Source: CAD feature listing. Evaluate the final solid. Frame: model axes, mm. Face numbers are marked on the shaded views. Coordinates: 2 decimals unless noted, no trailing zeros. Loops run counter-clockwise (first coordinate to the right, second up) from the corner with the lowest first, then second, coordinate; pieces in that order, holes last.
Item 1: Line query: probe 1 along Z at (x, y) = (0, -0.45); probe 2 along Z at (x, y) = (0, 78); probe 3 along Y at (x, z) = (20, 30.5). Output: solid intervals per line, ascending.
Item 2: Pull-direction query (Y, two-part tool) for the marked faces 1, 2 and 3; classes: +Y half, -Y half, draft (parallel to the pull), parting line (faces both ways), or undercut.
Item 3: Pin query (flat end, axial travel): pin 1 Ø12 at (x, z) = (-7, -14.5) entering from +Y; pin 2 Ø5 at (x, y) = (17, 91) entering from +Z; pin 3 Ø3 at (x, y) = (-14, 119) entering from +Z; pin 4 Ø1.5 at (y, z) = (69, -17) entering from +X. Return the tip coordinate at first contact, or that it passes through.
Item 4: Section query A-A, the plane z = 0. Return the cut outline in (x, y).
Item 5: Section query B-B, the plane x = 0. Return the cut outline in (y, z).
Item 6: Section query D-D, the plane x = 33. Return the cut outline in (y, z), then the cut area to 3 significant figures.
Item 7: Section query C-C, the plane y = 74. Return the cut outline in (x, z), then the cut area to 3 significant figures.
```python
from build123d import *

# Parameters (mm, degrees)
F0_R     = 40
F0_R_2   = 28
F0_R_3   = 25.5
F1_DEPTH = 2.5
F2_DEPTH = 160


with BuildPart() as f1:
    # F0 (on Front) → F1 (new body)
    with BuildSketch(Plane.XZ):
        Circle(F0_R)
        with BuildLine():
            ThreePointArc((24.4501319139, 21.4112365218), (30.4210394892, 11.4372355226), (32.5, 0))
            ThreePointArc((32.5, 0), (30.4210394892, -11.4372355226), (24.4501319139, -21.4112365218))
            ThreePointArc((24.4501319139, -21.4112365218), (24.9534304363, -22.1254580507), (25.1309703886, -22.9809703886))
            ThreePointArc((25.1309703886, -22.9809703886), (23.7707716884, -24.9806488394), (21.4112365218, -24.4501319139))
            ThreePointArc((21.4112365218, -24.4501319139), (0, -32.5), (-21.4112365218, -24.4501319139))
            ThreePointArc((-21.4112365218, -24.4501319139), (-24.5012499681, -24.5012499681), (-24.4501319139, -21.4112365218))
            ThreePointArc((-24.4501319139, -21.4112365218), (-32.5, 0), (-24.4501319139, 21.4112365218))
            ThreePointArc((-24.4501319139, 21.4112365218), (-24.5012499681, 24.5012499681), (-21.4112365218, 24.4501319139))
            ThreePointArc((-21.4112365218, 24.4501319139), (0, 32.5), (21.4112365218, 24.4501319139))
            ThreePointArc((21.4112365218, 24.4501319139), (23.7707716884, 24.9806488394), (25.1309703886, 22.9809703886))
            ThreePointArc((25.1309703886, 22.9809703886), (24.9534304363, 22.1254580507), (24.4501319139, 21.4112365218))
        make_face(mode=Mode.SUBTRACT)
        with BuildLine():
            ThreePointArc((24.4501319139, -21.4112365218), (30.4210394892, -11.4372355226), (32.5, 0))
            ThreePointArc((32.5, 0), (30.4210394892, 11.4372355226), (24.4501319139, 21.4112365218))
            ThreePointArc((24.4501319139, 21.4112365218), (21.460690809, 21.460690809), (21.4112365218, 24.4501319139))
            ThreePointArc((21.4112365218, 24.4501319139), (0, 32.5), (-21.4112365218, 24.4501319139))
            ThreePointArc((-21.4112365218, 24.4501319139), (-20.9812919377, 23.7707716884), (-20.8309703886, 22.9809703886))
            ThreePointArc((-20.8309703886, 22.9809703886), (-22.1254580507, 21.0085103409), (-24.4501319139, 21.4112365218))
            ThreePointArc((-24.4501319139, 21.4112365218), (-32.5, 0), (-24.4501319139, -21.4112365218))
            ThreePointArc((-24.4501319139, -21.4112365218), (-22.1254580507, -21.0085103409), (-20.8309703886, -22.9809703886))
            ThreePointArc((-20.8309703886, -22.9809703886), (-20.9812919377, -23.7707716884), (-21.4112365218, -24.4501319139))
            ThreePointArc((-21.4112365218, -24.4501319139), (0, -32.5), (21.4112365218, -24.4501319139))
            ThreePointArc((21.4112365218, -24.4501319139), (21.460690809, -21.460690809), (24.4501319139, -21.4112365218))
        make_face()
        Circle(F0_R_2, mode=Mode.SUBTRACT)
        Circle(F0_R_2)
        Circle(F0_R_3, mode=Mode.SUBTRACT)
    extrude(amount=F1_DEPTH)

    # F0 (on Front) → F2 (join)
    with BuildSketch(Plane.XZ):
        Circle(F0_R_2)
        Circle(F0_R_3, mode=Mode.SUBTRACT)
    extrude(amount=-F2_DEPTH)


solid = f1.part
```
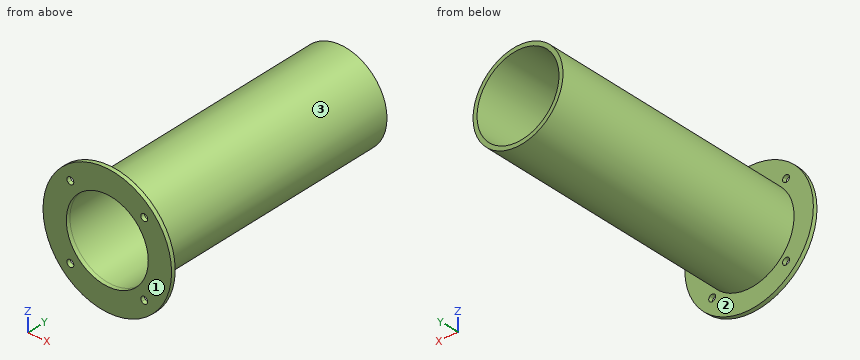
Verdict:
1. probe 1: z = -40 to -25.5, 25.5 to 40
1. probe 2: z = -28 to -25.5, 25.5 to 28
1. probe 3: y = -2.5 to 0
2. face 1: -Y half
2. face 2: +Y half
2. face 3: draft
3. pin 1: passes through
3. pin 2: stops at z = 23.95
3. pin 3: stops at z = 25.05
3. pin 4: stops at x = 22.8
4. outline: (-40, -2.5) - (-25.5, -2.5) - (-25.5, 160) - (-28, 160) - (-28, 0) - (-40, 0) - close; (25.5, -2.5) - (40, -2.5) - (40, 0) - (28, 0) - (28, 160) - (25.5, 160) - close
5. outline: (-2.5, -40) - (0, -40) - (0, -28) - (160, -28) - (160, -25.5) - (-2.5, -25.5) - close; (-2.5, 25.5) - (160, 25.5) - (160, 28) - (0, 28) - (0, 40) - (-2.5, 40) - close
6. outline: (-2.5, -22.61) - (0, -22.61) - (0, 22.61) - (-2.5, 22.61) - close
6. area: 113 mm2
7. outline: circle Ø56 at (0, 0); hole circle Ø51 at (0, 0)
7. area: 420 mm2
